from build123d import *

# Parameters (mm, degrees)
BOSS_EXTRUDE1_DEPTH = 19
CUT_EXTRUDE1_DEPTH  = 19
SKETCH6_R           = 3
CUT_EXTRUDE2_DEPTH  = 10
SKETCH7_R           = 0.5
CUT_EXTRUDE3_DEPTH  = 20


with BuildPart() as part:
    # Sketch2 → Boss-Extrude1 (new body)
    with BuildSketch(Plane.XY):
        Polygon((-50, -12.7), (50, -12.7), (50, 34.001988406), (86.488954477, 32.648136171), (79.389661188, -158.69164437), (-79.389661188, -158.69164437), (-86.488954477, 32.648136171), (-50, 34.001988406), align=None)
    extrude(amount=-BOSS_EXTRUDE1_DEPTH)

    # Sketch4 → Cut-Extrude1 (cut)
    with BuildSketch(Plane(origin=(0, 0, -19), x_dir=(-1, 0, 0), z_dir=(0, 0, -1))):
        Polygon((176.999986596, -116.887260719), (45, -111.989655964), (45, -158.69164437), (-45, -158.69164437), (-45, -111.989655964), (-160.814787096, -116.286740127), (-160.814787096, -226.328943165), (176.999986596, -226.328943165), align=None)
    extrude(amount=-CUT_EXTRUDE1_DEPTH, mode=Mode.SUBTRACT)

    # Sketch6 → Cut-Extrude2 (cut)
    with BuildSketch(Plane(origin=(0, -12.7, 0), x_dir=(1, 0, 0), z_dir=(0, 1, 0))):
        with Locations((35, 9.5)):
            Circle(SKETCH6_R)
        with Locations((-35, 9.5)):
            Circle(SKETCH6_R)
    extrude(amount=-CUT_EXTRUDE2_DEPTH, mode=Mode.SUBTRACT)

    # Sketch7 → Cut-Extrude3 (cut)
    with BuildSketch(Plane(origin=(0, 0, -19), x_dir=(-1, 0, 0), z_dir=(0, 0, -1))):
        with Locations((68.244477239, 33.325062289)):
            Circle(SKETCH7_R)
        with Locations((-68.244477239, 33.325062289)):
            Circle(SKETCH7_R)
    extrude(amount=-CUT_EXTRUDE3_DEPTH, mode=Mode.SUBTRACT)


solid = part.part
Can you work these out from the model? Positions are in its coordinate system, mm. A direction names the side the tool comes from. Give positions to 0.01 mm unless a question says otherwise; leave off trailing zeros. Loops run counter-clockwise (first coordinate to the right, second up) from the corner with the lowest first, then second, coordinate; pieces in that order, holes last. Notation, with made-up numbers: (52, -10.5) - (80, -10.5) arc R17 cw to (80, 20.5) - close; hole circle Ø7 at (-28.5, -9). An arc over 180 degrees is marked (long way). Answer as a JSON object with one key per item and string values.
Q1. Imagine slicing it at A-A on y = -10. Write out the boundary of the cut face in (x, z).
Geometry says:
{"outline": "(-84.91, -19) - (-50, -19) - (-50, 0) - (-84.91, 0) - close; (50, -19) - (84.91, -19) - (84.91, 0) - (50, 0) - close"}
Q2. If I drill on L1, parallel to Z at x = -35, y = -17; L2, parallel to X at y = -16.5, z = -9.5; L3, parallel to Y at x = -8.5, z = -8.75, over which ranges is the centre line in solid material (lowest first)?
Geometry says:
{"L1": "-19 to -12.5, -6.5 to 0", "L2": "-84.67 to -38, -32 to 32, 38 to 84.67", "L3": "-158.69 to -12.7"}
Q3. Imagine slicing it at D-D on y = -135.5. Write out the boundary of the cut face in (x, z), plus the area to 3 significant figures.
Geometry says:
{"outline": "(-45, -19) - (45, -19) - (45, 0) - (-45, 0) - close", "area": "1,710 mm²"}
Q4. If we mould it in two halves opening along Z, with no side actions, what happens to faces 6 (the flat face through (-63.29, -112.67, -9.63)), 7 (the flat face through (1, -61, -19)), 8 (the flat face through (35, -22.7, -10)), 9 (the flat face through (1, -61, 0))? For each: pulls with the +Z half, pulls with the -Z half, needs draft (parallel to the pull), parting line crosses it, or undercut.
Geometry says:
{"face 6": "needs draft", "face 7": "pulls with the -Z half", "face 8": "undercut", "face 9": "pulls with the +Z half"}
Q5. Imagine slicing it at C-C on z = -2.25. Write out the boundary of the cut face in (x, y).
Geometry says:
{"outline": "(-86.49, 32.65) - (-81.07, -113.33) - (-45, -111.99) - (-45, -158.69) - (45, -158.69) - (45, -111.99) - (81.07, -113.33) - (86.49, 32.65) - (68.74, 33.31) arc R0.5 cw to (67.74, 33.34) - (50, 34) - (50, -12.7) - (-50, -12.7) - (-50, 34) - (-67.74, 33.34) arc R0.5 cw to (-68.74, 33.31) - close"}
Q6. Will these pins go through, and if not, where does the flat tip stop? P1, Ø3, axis at x = 63.5, z = -10.5, coming from the +Y side; P2, Ø9.5, axis at x = -9, z = -7.5, coming from the +Y side; P3, Ø10, axis at y = -24.5, z = -17, coming from the -X side.
Geometry says:
{"P1": "y = 33.56", "P2": "y = -12.7", "P3": "x = -84.55"}
Q7. Which directions (+Z, -Z, +X, -X, +Y, -Y) give clear straight access to the entire face, cutting with the end or side of a thin tool? Please do faces 1 (the flat face through (-1, -158.692, -10)), 2 (the flat face through (83.82, -39.32, -9.37)), 3 (the cylindrical face through (-38, -17.6, -9.6)), 4 (the flat face through (-1, -12.7, -9)), 5 (the flat face through (62.78, -112.65, -9.63)).
Geometry says:
{"face 1": "+Z, -Z, +X, -X, -Y", "face 2": "+Z, -Z, +X, -Y", "face 3": "+Y", "face 4": "+Z, -Z, +Y", "face 5": "+Z, -Z, -Y"}
Q8. Imagine slicing it at B-B on x = 35. Write out the boundary of the cut face in (y, z).
Geometry says:
{"outline": "(-158.69, -19) - (-12.7, -19) - (-12.7, -12.5) - (-22.7, -12.5) - (-22.7, -6.5) - (-12.7, -6.5) - (-12.7, 0) - (-158.69, 0) - close"}
